```python
from build123d import *

# Parameters (mm, degrees)
F0_R     = 3.175
F0_R_2   = 1.5875
F1_DEPTH = 3.048


with BuildPart() as f1:
    # F0 (on Front) → F1 (new body)
    with BuildSketch(Plane.XZ):
        with BuildLine():
            ThreePointArc((-9.5097297278, 100.1845862784), (-0.2696751221, 90.1242705795), (9.525, 99.6454522461))
            ThreePointArc((9.525, 99.6454522461), (9.5238201928, 99.7953653394), (9.5202810634, 99.9452412949))
            ThreePointArc((9.5202810634, 99.9452412949), (0.1197887221, 109.1696989702), (-9.5097297278, 100.1845862784))
        make_face()
        with Locations((0, 99.6454522461)):
            Circle(F0_R, mode=Mode.SUBTRACT)
        with BuildLine():
            ThreePointArc((9.5202810634, 99.9452412949), (9.5238201928, 99.7953653394), (9.525, 99.6454522461))
            ThreePointArc((9.525, 99.6454522461), (-0.2696751221, 90.1242705795), (-9.5097297278, 100.1845862784))
            Line((-9.5097297278, 100.1845862784), (-15.5077525398, 39.540336068))
            ThreePointArc((-15.5077525398, 39.540336068), (0.9122205372, 51.9942212422), (15.7948542636, 37.7386263705))
            Line((15.7948542636, 37.7386263705), (9.5202810634, 99.9452412949))
        make_face()
        with Locations((-1.5875, 86.6684019566)):
            Circle(F0_R_2, mode=Mode.SUBTRACT)
        with BuildLine():
            Line((15.2064214472, 31.5869029408), (15.7948542636, 37.7386263705))
            ThreePointArc((15.7948542636, 37.7386263705), (0.9122205372, 51.9942212422), (-15.5077525398, 39.540336068))
            Line((-15.5077525398, 39.540336068), (-15.8723283432, 35.854217003))
            Line((-15.8723283432, 35.854217003), (-15.610768577, 33.2610927966))
            ThreePointArc((-15.610768577, 33.2610927966), (-0.8611632068, 20.2938270003), (15.2064214472, 31.5869029408))
        make_face()
        with Locations((0, 36.1454522461)):
            Circle(F0_R, mode=Mode.SUBTRACT)
        with BuildLine():
            ThreePointArc((15.875, 36.1454522461), (15.8549509056, 36.9430466182), (15.7948542636, 37.7386263705))
            Line((15.7948542636, 37.7386263705), (15.2064214472, 31.5869029408))
            ThreePointArc((15.2064214472, 31.5869029408), (15.7069660577, 33.8417937943), (15.875, 36.1454522461))
        make_face()
        with BuildLine():
            Line((-15.8723283432, 35.854217003), (-15.5077525398, 39.540336068))
            ThreePointArc((-15.5077525398, 39.540336068), (-15.797918771, 37.7079462474), (-15.8723283432, 35.854217003))
        make_face()
        with BuildLine():
            Line((11.2344941696, -9.9372905003), (15.2064214472, 31.5869029408))
            ThreePointArc((15.2064214472, 31.5869029408), (-0.8611632068, 20.2938270003), (-15.610768577, 33.2610927966))
            Line((-15.610768577, 33.2610927966), (-9.5217535723, -27.1058835037))
            ThreePointArc((-9.5217535723, -27.1058835037), (0.1243427206, -17.8303593954), (9.525, -27.3545477539))
            ThreePointArc((9.525, -27.3545477539), (6.9227046125, -33.8968551334), (0.5377483785, -36.8643559371))
            Line((0.5377483785, -36.8643559371), (44.6741512192, -35.6174676663))
            ThreePointArc((44.6741512192, -35.6174676663), (36.5127135943, -27.6249029998), (44.7905380327, -19.7529415784))
            Line((44.7905380327, -19.7529415784), (18.8074885558, -18.6371783145))
            ThreePointArc((18.8074885558, -18.6371783145), (13.1519949788, -15.9141403429), (11.2344941696, -9.9372905003))
        make_face()
        with BuildLine():
            Line((-15.610768577, 33.2610927966), (-15.8723283432, 35.854217003))
            ThreePointArc((-15.8723283432, 35.854217003), (-15.7948542636, 34.5522781217), (-15.610768577, 33.2610927966))
        make_face()
        with BuildLine():
            ThreePointArc((9.525, -27.3545477539), (0.1243427206, -17.8303593954), (-9.5217535723, -27.1058835037))
            ThreePointArc((-9.5217535723, -27.1058835037), (-6.8225417545, -34.0012423466), (0, -36.8795477539))
            Line((0, -36.8795477539), (0.5377483785, -36.8643559371))
            ThreePointArc((0.5377483785, -36.8643559371), (6.9227046125, -33.8968551334), (9.525, -27.3545477539))
        make_face()
        with Locations((0, -27.3545477539)):
            Circle(F0_R, mode=Mode.SUBTRACT)
        with BuildLine():
            Line((0.5377483785, -36.8643559371), (0, -36.8795477539))
            ThreePointArc((0, -36.8795477539), (0.2689814631, -36.8757490422), (0.5377483785, -36.8643559371))
        make_face()
        with BuildLine():
            ThreePointArc((52.3875, -27.6831332594), (50.1817940858, -22.1921913723), (44.7905380327, -19.7529415784))
            ThreePointArc((44.7905380327, -19.7529415784), (36.5127135943, -27.6249029998), (44.6741512192, -35.6174676663))
            ThreePointArc((44.6741512192, -35.6174676663), (50.1413577709, -33.2159763779), (52.3875, -27.6831332594))
        make_face()
        with Locations((44.45, -27.6831332594)):
            Circle(F0_R, mode=Mode.SUBTRACT)
    extrude(amount=F1_DEPTH)


solid = f1.part
```
For this review, take the finished solid that the model builds, in its own axes (mm). A direction names the side the tool comes from. Round coordinates to 2 decimals unless told otherwise and drop trailing zeros. Write each loop counter-clockwise with the first axis right and the second up, starting at its lowest first coordinate (ties: lowest second). Pieces come first, ordered by that corner, then holes. Notation, with made-up numbers: (28, -26.5) -> (72, -26.5) arc R5 cw to (72, -19.5) -> close; hole circle Ø3 at (10.5, 65). An arc over 180 degrees is marked (long way). One line per question, with ' | ' between items. Start each with the question number.
1) Add section A-A (x = 43). Write out the cut boundary in (y, z), and give its area (3 significant figures).
2) Mouldability with a two-part tool opening along Z and no side actions: class faces 1 (the cylindrical face through (13.21, -1.5, -15.98)), 2 (the flat face through (31.981, -1.503, -19.203)), 3 (the flat face through (3, 0, 21)) as +Z half, -Z half, draft (parallel to the pull), parting line (faces both ways), or undercut.
3) For pin 1 Ø10 at (x, z) = (44.45, -27.68) entering from +Y; pin 2 Ø1 at (x, y) = (30, -0.5) entering from -Z, all flat-tipped, find the tip position at first contact; note any pin that passes through.
4) Add section D-D (z = -17). Write out the cut boundary in (x, y).
5) Wall thickness on line 1 along Z through (x, y) = (44.45, -1.6); line 2 along Z through (x, y) = (43, -1.65); line 3 along X through (y, z) = (-2.5, 44): over which ranges is each line inside the solid? List them lowest first.
6) Add section C-C (x = 13). Write out the cut boundary in (y, z), and give its area (3 significant figures).
7) Machinability: for faces 4 (the cylindrical face through (-1.93, -1.5, 85.12)), 5 (the flat face through (13.193, -1.503, 10.534)), which of the approach directions +Z, -Z, +X, -X, +Y, -Y give a long, thin tool a straight path to every point of the face, cutting with its end or side? Answer none if there is none.
8) Add section B-B (y = -1.6). Count the separate pieces of the cut face and the enclosed holes in it, and give its area (3 significant figures).
Reported:
1) outline: (-3.05, -35.66) -> (0, -35.66) -> (0, -30.51) -> (-3.05, -30.51) -> close; (-3.05, -24.86) -> (0, -24.86) -> (0, -19.68) -> (-3.05, -19.68) -> close | area: 31.5 mm²
2) face 1: undercut | face 2: +Z half | face 3: draft
3) pin 1: stops at y = 0 | pin 2: stops at z = -36.05
4) outline: (-10.54, -3.05) -> (14.31, -3.05) -> (14.31, 0) -> (-10.54, 0) -> close
5) line 1: z = -35.62 to -30.86, -24.51 to -19.74 | line 2: z = -35.66 to -30.51, -24.86 to -19.68 | line 3: x = -15.07 to 15.16
6) outline: (-3.05, -36.51) -> (0, -36.51) -> (0, -15.73) -> (-3.05, -15.73) -> close; (-3.05, 8.52) -> (0, 8.52) -> (0, 65.45) -> (-3.05, 65.45) -> close | area: 237 mm²
7) face 4: +Y, -Y | face 5: +X, +Y, -Y
8) separate pieces: 1 | enclosed holes: 5 | area: 4,100 mm²
